Geometry check sheet. Reference: drawing and pictorial views, mm from the part's lowest x, y, z. A direction names the side the tool comes from. Round coordinates to 2 decimals unless told otherwise and drop trailing zeros. Write each loop counter-clockwise with the first axis right and the second up, starting at its lowest first coordinate (ties: lowest second). Pieces come first, ordered by that corner, then holes. Notation, with made-up numbers: M 22,51.5 L 64,51.5 A32 cw 64,84.5 Z; hole C 63.25,-30.75 d5. An arc over 180 degrees is marked long. Put each result on its own line as item: value. Start each with the question number.
(1) Section check D-D on x = 9.5. Record the cut outline in (y, z) (1 decimal).
(2) Gauge pin test, flat ends, axial feed: pin 1 (5 mm diameter, centred on x = 19.5, y = 8.5, fed in from -Z); pin 2 (4 mm diameter, centred on x = 22.5, y = 18, fed in from +Z); pin 3 (2 mm diameter, centred on x = 24, y = 15.5, fed in from +Z). Record the tip position at first contact, or that the pin passes through.
(3) Section check B-B on y = 6. Record the cut outline in (x, z).
(4) Section check A-A on x = 17.25. Record the cut outline in (y, z).
(5) Tool access check on the marked faces 1, 2 and 3. Record the directions out of +Z, -Z, +X, -X, +Y, -Y that give a thin tool (end or side, any length) a straight path to the whole face; none if there is none.
(6) Material ranges on probe 1 along Y at (x, z) = (25.5, 13.75) (1 decimal); probe 2 along X at (y, z) = (17.75, 3.5); probe 3 along Y at (x, z) = (26.75, 11.25) (1 decimal), recorded low to high.
(7) Section check C-C on z = 18.25. Record the cut outline in (x, y) (1 decimal).
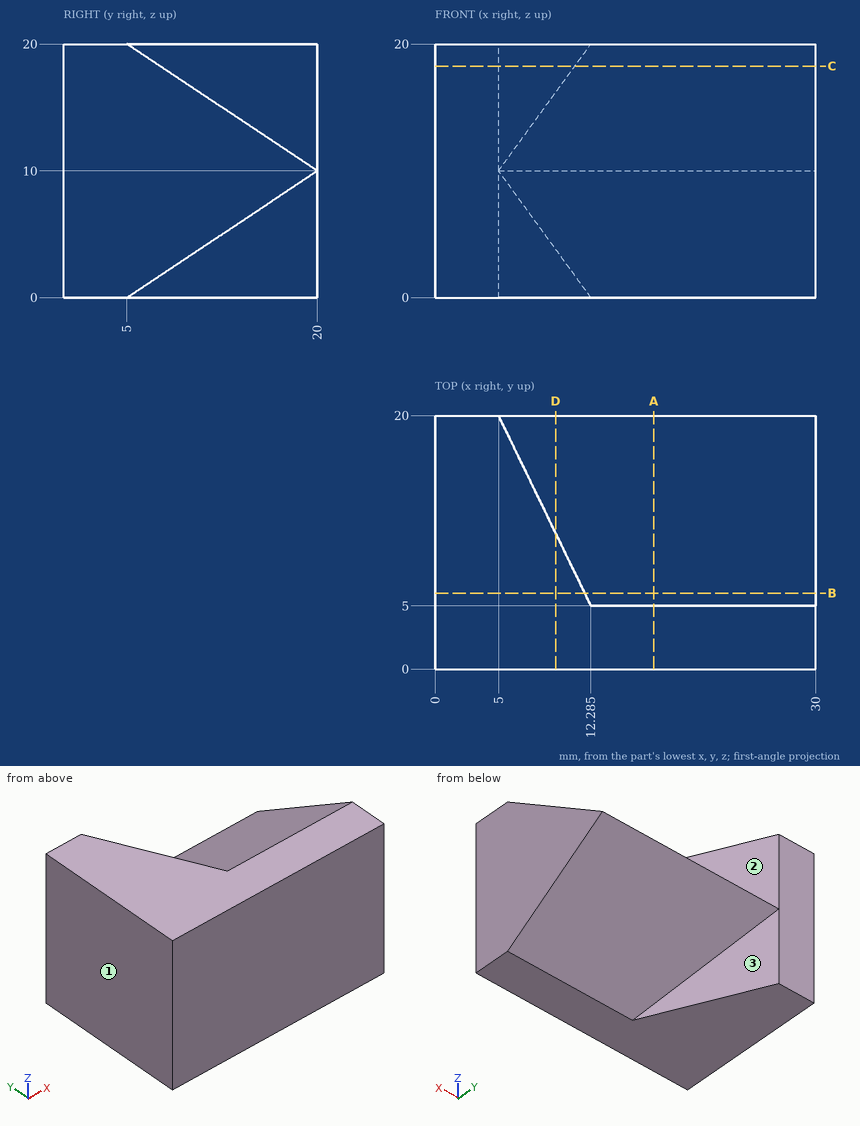
Answers follow:
1. outline: M 0,0 L 10.7,0 L 10.7,3.8 L 20,10 L 10.7,16.2 L 10.7,20 L 0,20 Z
2. pin 1: stops at z = 0.67
2. pin 2: stops at z = 12.67
2. pin 3: stops at z = 13.67
3. outline: M 0,0 L 11.8,0 L 11.8,0.67 L 30,0.67 L 30,19.33 L 11.8,19.33 L 11.8,20 L 0,20 Z
4. outline: M 0,0 L 5,0 L 20,10 L 5,20 L 0,20 Z
5. face 1: +Z, -Z, -X, +Y, -Y
5. face 2: +Z, +X, +Y
5. face 3: -Z, +X, +Y
6. probe 1: y = 0 to 14.4
6. probe 2: x = 0 to 6.09
6. probe 3: y = 0 to 18.1
7. outline: M 0,0 L 30,0 L 30,7.6 L 11,7.6 L 5,20 L 0,20 Z
